CAD build for the part. Positions are in the model's coordinates, mm. A direction names the side the tool comes from. Round coordinates to 2 decimals unless told otherwise and drop trailing zeros. Loops run counter-clockwise (first coordinate to the right, second up) from the corner with the lowest first, then second, coordinate; pieces in that order, holes last. Notation, with made-up numbers: (-10.75, 78.5) - (0.25, 78.5) arc R12 cw to (0.25, 95.5) - close; hole circle Ø10 at (-3.75, -16.75). An arc over 180 degrees is marked (long way). Use one line per item in the form item = value.
from build123d import *

# Parameters (mm, degrees)
SKETCH1_R           = 5.334
BOSS_EXTRUDE2_DEPTH = 0.0254
SKETCH2_R           = 2.794
BOSS_EXTRUDE4_DEPTH = 7.62
SKETCH3_R           = 2.794
BOSS_EXTRUDE5_DEPTH = 0.2286
BOSS_EXTRUDE5_TAPER = 84.999999999


with BuildPart() as part:
    # Sketch1 → Boss-Extrude2 (new body)
    with BuildSketch(Plane(origin=(0, 0, 0), x_dir=(1, 0, 0), z_dir=(0, 1, 0))):
        with Locations(Location((0, 0, 0), (0, 0, 270))):
            Circle(SKETCH1_R)
    extrude(amount=BOSS_EXTRUDE2_DEPTH)

    # Sketch2 → Boss-Extrude4 (add)
    with BuildSketch(Plane(origin=(0, 0.0254, 0), x_dir=(1, 0, 0), z_dir=(0, 1, 0))):
        with Locations(Location((0, 0, 0), (0, 0, 90))):
            Circle(SKETCH2_R)
    extrude(amount=BOSS_EXTRUDE4_DEPTH)

    # Sketch3 → Boss-Extrude5 (add)
    with BuildSketch(Plane(origin=(0, 7.6454, 0), x_dir=(1, 0, 0), z_dir=(0, 1, 0))):
        with Locations(Location((0, 0, 0), (0, 0, 90))):
            Circle(SKETCH3_R)
    extrude(amount=BOSS_EXTRUDE5_DEPTH, taper=BOSS_EXTRUDE5_TAPER)


solid = part.part
1) Slice it at B-B (y = 5.75). Write the cut outline in (x, z).
Report:
outline = circle Ø5.59 at (0, 0)
2) Drill centre lines: probe 1 along Y at (x, z) = (-0.75, -2.25); probe 2 along X at (y, z) = (2, 2); probe 3 along Z at (x, y) = (-1, 7.25). Where is each one in solid material? Low to high.
Report:
probe_1 = 0 to 7.68
probe_2 = -1.95 to 1.95
probe_3 = -2.61 to 2.61
3) Flat gauge pins, fed straight in: pin 1 (3 mm diameter, centred on y = 2.5, z = 2.5, fed in from +X); pin 2 (2 mm diameter, centred on x = 3.5, y = 2, fed in from -Z); pin 3 (4 mm diameter, centred on y = 6.5, z = -2, fed in from +X); pin 4 (5.5 mm diameter, centred on x = 2.5, z = 1.5, fed in from +Y). Where does each tip first touch, or does it go through?
Report:
pin_1 = 2.61
pin_2 = -1.25
pin_3 = 2.79
pin_4 = 7.87
4) Tool access for faces 1 (the cylindrical face through (2.728, 3.782, 0.606)), 2 (the flat face through (0, 0, 0)): list every direction of +Z, -Z, +X, -X, +Y, -Y with a clear straight run to the whole face (end or side of a thin tool).
Report:
face_1 = +Y
face_2 = +Z, -Z, +X, -X, -Y
